Read the model definition and answer for the solid it produces. Units are mm, in the model's axes. Face numbers are marked on the shaded views. A direction names the side the tool comes from. Give positions to 0.01 mm unless a question says otherwise; leave off trailing zeros. Order: outer loops, then holes, each group sorted by start corner. A loop starts at its lowest first (then second) coordinate and runs counter-clockwise, first axis right, second up. Notation, with made-up numbers: (87.5, 1) - (110.5, 1) arc R27 cw to (110.5, 36) - close; hole circle Ø4 at (27.5, -3). An arc over 180 degrees is marked (long way). Use a Markdown table: item, result. Add a question column.
1. Flat-ended cylindrical pins translate along their axes: P1, Ø3, axis at y = 16, z = -15, coming from the +X side; P2, Ø1.5, axis at y = -9, z = 2, coming from the +X side; P3, Ø16, axis at x = 21, z = 1.5, coming from the +Y side; P4, Ø8, axis at y = 7.5, z = 0, coming from the -X side. Find the tip coordinate at first contact, or state that the pin passes through.
2. A cutting plane is placed at B-B on x = 37.5. Determine the outline of the cut face in (y, z), and give its area (3 significant figures).
3. For a pull along X with two mould halves and no side action, classify the marked faces 5, 6 and 7 as released by +X, released by -X, zero draft, split by the parting line, or undercut.
4. A cutting plane is placed at C-C on y = -5. Determine the outline of the cut face in (x, z).
5. Which of the six approach directions +Z, -Z, +X, -X, +Y, -Y give full straight-line access (tool end or side, diameter ignored) to the marked faces 1, 2, 3 and 4?
6. Consider L1, parallel to X at y = 14, z = -9.5; L2, parallel to Y at x = 7.5, z = 7; L3, parallel to Y at x = 42.5, z = -0.5. Determine where each line is inside the solid, lowest interval first.
7. A cutting plane is placed at A-A on y = 0. Determine the outline of the cut face in (x, z), and give its area (3 significant figures).
8. A cutting plane is placed at D-D on x = 16.5. Determine the outline of the cut face in (y, z).
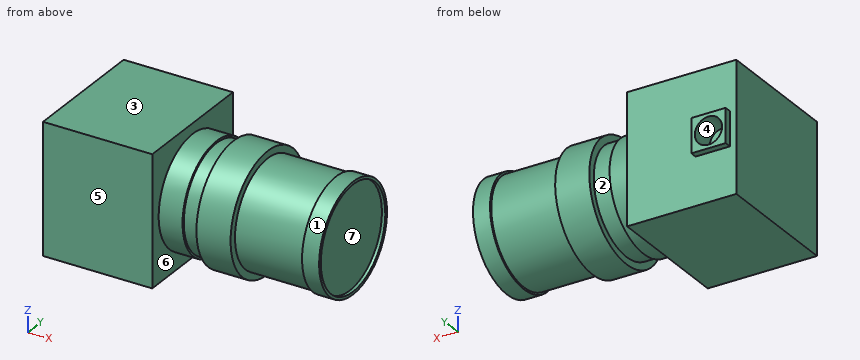
```python
from build123d import *

# Parameters (mm, degrees)
SKETCH1_W           = 38
SKETCH1_H           = 38
BOSS_EXTRUDE1_DEPTH = 32
SKETCH2_R           = 16
BOSS_EXTRUDE2_DEPTH = 47
SKETCH3_W           = 10.074074074
SKETCH3_H           = 10
SKETCH3_R           = 4
BOSS_EXTRUDE3_DEPTH = 2
CUT_EXTRUDE1_START  = -5
SKETCH3_2_R         = 4
CUT_EXTRUDE1_DEPTH  = 5
CUT_EXTRUDE2_START  = -25
SKETCH4_R           = 16
SKETCH4_R_2         = 15.412875145
CUT_EXTRUDE2_DEPTH  = 20
BOSS_EXTRUDE4_START = -35
SKETCH5_R           = 17.5
SKETCH5_R_2         = 16
BOSS_EXTRUDE4_DEPTH = 10
CUT_EXTRUDE3_START  = -40
SKETCH4_2_R         = 16
SKETCH4_2_R_2       = 15.412875145
CUT_EXTRUDE3_DEPTH  = 5
SKETCH6_R           = 15.197678489
CUT_EXTRUDE4_DEPTH  = 1


with BuildPart() as part:
    # Sketch1 → Boss-Extrude1 (new body)
    with BuildSketch(Plane(origin=(0, 0, 0), x_dir=(0, 0, -1), z_dir=(1, 0, 0))):
        Rectangle(SKETCH1_W, SKETCH1_H)
    extrude(amount=BOSS_EXTRUDE1_DEPTH)

    # Sketch2 → Boss-Extrude2 (add)
    with BuildSketch(Plane(origin=(32, 0, 0), x_dir=(0, 0, -1), z_dir=(1, 0, 0))):
        Circle(SKETCH2_R)
    extrude(amount=BOSS_EXTRUDE2_DEPTH)

    # Sketch3 → Boss-Extrude3 (add)
    with BuildSketch(Plane(origin=(0, 19, 0), x_dir=(1, 0, 0), z_dir=(0, 1, 0))):
        with Locations((6.924898334, 0)):
            Rectangle(SKETCH3_W, SKETCH3_H)
        with Locations(Location((6.924898334, 0, 0), (0, 0, 270))):
            Circle(SKETCH3_R, mode=Mode.SUBTRACT)
    extrude(amount=BOSS_EXTRUDE3_DEPTH)

    # Sketch3_2 → Cut-Extrude1 (cut)
    with BuildSketch(Plane(origin=(0, 19, 0), x_dir=(1, 0, 0), z_dir=(0, 1, 0)).offset(CUT_EXTRUDE1_START)):
        with Locations(Location((6.924898334, 0, 0), (0, 0, 270))):
            Circle(SKETCH3_2_R)
    extrude(amount=CUT_EXTRUDE1_DEPTH, mode=Mode.SUBTRACT)

    # Sketch4 → Cut-Extrude2 (cut)
    with BuildSketch(Plane(origin=(79, 0, 0), x_dir=(0, 0, -1), z_dir=(1, 0, 0)).offset(CUT_EXTRUDE2_START)):
        Circle(SKETCH4_R)
        Circle(SKETCH4_R_2, mode=Mode.SUBTRACT)
    extrude(amount=CUT_EXTRUDE2_DEPTH, mode=Mode.SUBTRACT)

    # Sketch5 → Boss-Extrude4 (add)
    with BuildSketch(Plane(origin=(79, 0, 0), x_dir=(0, 0, -1), z_dir=(1, 0, 0)).offset(BOSS_EXTRUDE4_START)):
        Circle(SKETCH5_R)
        Circle(SKETCH5_R_2, mode=Mode.SUBTRACT)
    extrude(amount=BOSS_EXTRUDE4_DEPTH)

    # Sketch4_2 → Cut-Extrude3 (cut)
    with BuildSketch(Plane(origin=(79, 0, 0), x_dir=(0, 0, -1), z_dir=(1, 0, 0)).offset(CUT_EXTRUDE3_START)):
        Circle(SKETCH4_2_R)
        Circle(SKETCH4_2_R_2, mode=Mode.SUBTRACT)
    extrude(amount=CUT_EXTRUDE3_DEPTH, mode=Mode.SUBTRACT)

    # Sketch6 → Cut-Extrude4 (cut)
    with BuildSketch(Plane(origin=(79, 0, 0), x_dir=(0, 0, -1), z_dir=(1, 0, 0))):
        Circle(SKETCH6_R)
    extrude(amount=-CUT_EXTRUDE4_DEPTH, mode=Mode.SUBTRACT)


solid = part.part
```
Output values:
| question | item | result |
|---|---|---|
| 1 | P1 | x = 32 |
| 1 | P2 | x = 78 |
| 1 | P3 | y = 19 |
| 1 | P4 | x = 0 |
| 2 | outline | circle Ø32 at (0, 0) |
| 2 | area | 804 mm² |
| 3 | face 5 | zero draft |
| 3 | face 6 | undercut |
| 3 | face 7 | released by +X |
| 4 | outline | (0, -19) - (32, -19) - (32, -15.2) - (39, -15.2) - (39, -14.58) - (44, -14.58) - (44, -16.77) - (54, -16.77) - (54, -14.58) - (74, -14.58) - (74, -15.2) - (79, -15.2) - (79, -14.35) - (78, -14.35) - (78, 14.35) - (79, 14.35) - (79, 15.2) - (74, 15.2) - (74, 14.58) - (54, 14.58) - (54, 16.77) - (44, 16.77) - (44, 14.58) - (39, 14.58) - (39, 15.2) - (32, 15.2) - (32, 19) - (0, 19) - close |
| 5 | face 1 | +X |
| 5 | face 2 | none |
| 5 | face 3 | +Z, +X, -X, +Y, -Y |
| 5 | face 4 | +Y |
| 6 | L1 | 0 to 32, 44 to 54 |
| 6 | L2 | -19 to 19 |
| 6 | L3 | -15.4 to 15.4 |
| 7 | outline | (0, -19) - (32, -19) - (32, -16) - (39, -16) - (39, -15.41) - (44, -15.41) - (44, -17.5) - (54, -17.5) - (54, -15.41) - (74, -15.41) - (74, -16) - (79, -16) - (79, -15.2) - (78, -15.2) - (78, 15.2) - (79, 15.2) - (79, 16) - (74, 16) - (74, 15.41) - (54, 15.41) - (54, 17.5) - (44, 17.5) - (44, 15.41) - (39, 15.41) - (39, 16) - (32, 16) - (32, 19) - (0, 19) - close |
| 7 | area | 2,690 mm² |
| 8 | outline | (-19, -19) - (19, -19) - (19, 19) - (-19, 19) - close |
